from build123d import *

# Parameters (mm, degrees)
FLANGE_SKETCH_R      = 3
FLANGE_EXTRUDE_DEPTH = 0.5
JOINT_SKETCH_R       = 2
JOINT_EXTRUDE_DEPTH  = 3.4
HOLE_SKETCH_R        = 1
HOLE_EXTRUDE_DEPTH   = 9.879189152


with BuildPart() as part:
    # Flange Sketch → Flange Extrude (new, symmetric)
    with BuildSketch(Plane.XY):
        Circle(FLANGE_SKETCH_R)
    extrude(amount=FLANGE_EXTRUDE_DEPTH, both=True)

    # Joint Sketch → Joint Extrude (add)
    with BuildSketch(Plane.XY.offset(0.5)):
        Circle(JOINT_SKETCH_R)
    joint_extrude = extrude(amount=JOINT_EXTRUDE_DEPTH)

    # Joint Mirror: Joint Extrude across plane
    add(joint_extrude.mirror(Plane.XY))

    # Hole Sketch → Hole Extrude (cut, through all)
    with BuildSketch(Plane.XY.offset(3.9)):
        Circle(HOLE_SKETCH_R)
    extrude(amount=-HOLE_EXTRUDE_DEPTH, mode=Mode.SUBTRACT)


solid = part.part
Source: CAD feature listing. Evaluate the final solid. Frame: model axes, mm. A direction names the side the tool comes from. Give positions to 0.01 mm unless a question says otherwise; leave off trailing zeros. Write each loop counter-clockwise with the first axis right and the second up, starting at its lowest first coordinate (ties: lowest second). Pieces come first, ordered by that corner, then holes. Notation, with made-up numbers: M 48.5,47.25 L 63.5,47.25 A22 cw 63.5,60.25 Z; hole C 21.5,-9.5 d6. An arc over 180 degrees is marked long. Return JSON: item names as keys, results as strings. Group by question number.
1) Cut plane D-D, the plane x = 1.15. Output: boundary loops of the cut face in (y, z), plus the area to 3 significant figures.
2) Set-up query: faces 1 (the face through (0, -2, 2)), 2 (the face through (1, -1, -3.9)), 3 (the face through (1, -2, -0.5)). Return all of +Z, -Z, +X, -X, +Y, -Y with unobstructed straight access to the full face (end or side cutting, diameter ignored); none if empty.
3) Pin query (flat end, axial travel): P1, Ø3, axis at y = 2, z = -1.5, coming from the -X side; P2, Ø3, axis at y = -1.5, z = 1.5, coming from the -X side; P3, Ø1.5, axis at y = 0.5, z = 3, coming from the +X side. Return the tip coordinate at first contact, or that it passes through.
4) Pull-direction query (Y, two-part tool) for faces 4 (the face through (0, -2, -2)), 5 (the face through (1, -1, 3.9)), 6 (the face through (0, -1, 0)); classes: pulls with the +Y half, pulls with the -Y half, needs draft (parallel to the pull), parting line crosses it, or undercut.
5) Material intervals for line 1 along Y through (x, z) = (0, -1); line 2 along Z through (x, y) = (2.6, -0.25); line 3 along X through (y, z) = (-0.9, 3.25), sorted ascending. Write a range as [from, to].
6) Cut plane C-C, the plane z = -2. Output: boundary loops of the cut face in (x, y), plus the area to 3 significant figures.
7) Cut plane A-A, the plane y = 0. Output: boundary loops of the cut face in (x, z).
Recorded:
{
 "1": {"outline": "M -2.77,-0.5 L -1.64,-0.5 L -1.64,-3.9 L 1.64,-3.9 L 1.64,-0.5 L 2.77,-0.5 L 2.77,0.5 L 1.64,0.5 L 1.64,3.9 L -1.64,3.9 L -1.64,0.5 L -2.77,0.5 Z", "area": "27.8 mm²"},
 "2": {"face 1": "+Z", "face 2": "-Z, +X, -X, +Y, -Y", "face 3": "-Z"},
 "3": {"P1": "stops at x = -2.87", "P2": "stops at x = -2.98", "P3": "stops at x = 2"},
 "4": {"face 4": "parting line crosses it", "face 5": "needs draft", "face 6": "undercut"},
 "5": {"line 1": "y = [-2, -1], [1, 2]", "line 2": "z = [-0.5, 0.5]", "line 3": "x = [-1.79, -0.44], [0.44, 1.79]"},
 "6": {"outline": "C 0,0 d4; hole C 0,0 d2", "area": "9.42 mm²"},
 "7": {"outline": "M -3,-0.5 L -2,-0.5 L -2,-3.9 L -1,-3.9 L -1,3.9 L -2,3.9 L -2,0.5 L -3,0.5 Z; M 1,-3.9 L 2,-3.9 L 2,-0.5 L 3,-0.5 L 3,0.5 L 2,0.5 L 2,3.9 L 1,3.9 Z"}
}
